```python
from build123d import *

# Parameters (mm, degrees)
SKETCH1_R           = 1.5
BOSS_EXTRUDE1_DEPTH = 3.18
SKETCH2_R           = 1.5
CUT_EXTRUDE1_DEPTH  = 10


with BuildPart() as part:
    # Sketch1 → Boss-Extrude1 (new body)
    with BuildSketch(Plane.XY):
        Polygon((-203.18, 50), (-203.18, 12.5), (-200, 12.5), (-200, 1.5), (-196, 1.5), (-196, 4.5), (-193, 4.5), (-193, 1.5), (-190.18, 1.5), (-190.18, -1.5), (-193, -1.5), (-193, -4.5), (-196, -4.5), (-196, -1.5), (-200, -1.5), (-200, -12.5), (-203.18, -12.5), (-203.18, -50), (-12.5, -50), (-12.5, -53.18), (12.5, -53.18), (12.5, -50), (200, -50), (200, -75), (265.68, -75), (265.68, -78.18), (290.68, -78.18), (290.68, -75), (356.36, -75), (356.36, -12.5), (353.18, -12.5), (353.18, -1.5), (349.18, -1.5), (349.18, -4.5), (346.18, -4.5), (346.18, -1.5), (343.36, -1.5), (343.36, 1.5), (346.18, 1.5), (346.18, 4.5), (349.18, 4.5), (349.18, 1.5), (353.18, 1.5), (353.18, 12.5), (356.36, 12.5), (356.36, 75), (290.68, 75), (290.68, 78.18), (265.68, 78.18), (265.68, 75), (200, 75), (200, 50), (12.5, 50), (12.5, 53.18), (-12.5, 53.18), (-12.5, 50), align=None)
        with Locations(Location((0, -51.59, 0), (0, 0, 180))):
            Circle(SKETCH1_R, mode=Mode.SUBTRACT)
        with Locations(Location((0, 51.59, 0), (0, 0, 180))):
            Circle(SKETCH1_R, mode=Mode.SUBTRACT)
        with Locations(Location((278.18, -76.59, 0), (0, 0, 180))):
            Circle(SKETCH1_R, mode=Mode.SUBTRACT)
        with Locations(Location((278.18, 76.59, 0), (0, 0, 180))):
            Circle(SKETCH1_R, mode=Mode.SUBTRACT)
    extrude(amount=BOSS_EXTRUDE1_DEPTH)

    # Sketch2 → Cut-Extrude1 (cut)
    with BuildSketch(Plane.XY.offset(3.18)):
        with Locations((284.68, -70)):
            Circle(SKETCH2_R)
        with Locations((271.68, -70)):
            Circle(SKETCH2_R)
    extrude(amount=-CUT_EXTRUDE1_DEPTH, mode=Mode.SUBTRACT)


solid = part.part
```
Geometry: final body of the model. Coordinates: model frame, mm. Round coordinates to 2 decimals unless told otherwise and drop trailing zeros. Order: outer loops, then holes, each group sorted by start corner. A loop starts at its lowest first (then second) coordinate and runs counter-clockwise, first axis right, second up. Notation, with made-up numbers: (-9, -12.75) -> (42, -12.75) arc R33 ccw to (42, 19.25) -> close; hole circle Ø3 at (62, -1.75). An arc over 180 degrees is marked (long way). Use one line per item in the form item = value. Start each with the question number.
1. Line query: probe 1 along X at (y, z) = (-70, 1.75); probe 2 along X at (y, z) = (-51.59, 1.1); probe 3 along X at (y, z) = (76.59, 1.65). Output: solid intervals per line, ascending.
2. Cut plane A-A (z = 0.9). Count the separate pieces of the cut face and the enclosed holes in it, then the cut area to 3 significant figures.
3. Cut plane B-B (x = 299). Return the cut outline in (y, z).
4. Cut plane C-C (x = -22). Return the cut outline in (y, z), then the cut area to 3 significant figures.
5. Pin query (flat end, axial travel): pin 1 Ø2 at (x, y) = (269, -10) entering from -Z; pin 2 Ø1.6 at (y, z) = (76, 1) entering from -X; pin 3 Ø1.6 at (x, z) = (354, 1.5) entering from -Y; pin 4 Ø1 at (x, z) = (-198.5, 1) entering from +Y. Return the tip coordinate at first contact, or that it passes through.
Solution:
q1.probe_1 = 200 to 270.18, 273.18 to 283.18, 286.18 to 356.36
q1.probe_2 = -12.5 to -1.5, 1.5 to 12.5, 200 to 356.36
q1.probe_3 = 265.68 to 276.68, 279.68 to 290.68
q2.separate_pieces = 1
q2.enclosed_holes = 6
q2.area = 63,800 mm^2
q3.outline = (-75, 0) -> (75, 0) -> (75, 3.18) -> (-75, 3.18) -> close
q4.outline = (-50, 0) -> (50, 0) -> (50, 3.18) -> (-50, 3.18) -> close
q4.area = 318 mm^2
q5.pin_1 = 0
q5.pin_2 = 265.68
q5.pin_3 = -75
q5.pin_4 = 50
